Check sheet for the modelled part. Datum: model origin and axes. Units: mm. A direction names the side the tool comes from. Give positions to 0.01 mm unless a question says otherwise; leave off trailing zeros. Loops run counter-clockwise (first coordinate to the right, second up) from the corner with the lowest first, then second, coordinate; pieces in that order, holes last. Notation, with made-up numbers: (22.5, 59.5) -> (78.5, 59.5) arc R32 ccw to (78.5, 91.5) -> close; hole circle Ø5 at (51, -34.75). An arc over 180 degrees is marked (long way). Answer as CSV lines item,"result". Start each with the question number.
(1) Material ranges on line 1 (X direction, y = 14.25, z = 0) (3 decimals); line 2 (Y direction, x = 21.5, z = 2.5); line 3 (Z direction, x = 4, y = 13), recorded low to high. Write a range as from..to.
(2) Section check A-A on z = 0. Enter the section's corners in (x, y) (3 decimals), plus the area to 3 significant figures.
(3) Release check for a two-part mould opening along Z. For faces 6 (the face through (-24, 20, 0)), 7 (the face through (3.3, 0, -3.3)), 8 (the face through (-3.99, 10.5, -2.07)) record: pulls with the +Z half, pulls with the -Z half, needs draft (parallel to the pull), parting line crosses it, or undercut.
(4) Section check D-D on y = 9.75. Enter the section's corners in (x, z) (3 decimals).
(5) Section check C-C on y = 19.5. Enter the section's corners in (x, z) (3 decimals).
(6) Section check B-B on x = 0. Enter the section's corners in (y, z) (3 decimals).
(7) Access from +Z, -Z, +X, -X, +Y, -Y to the whole of each face (thin tool, end or side, straight path). Record for faces 1 (the face through (-0.31, 19.78, -12.17)), 2 (the face through (11.5, 9.15, -2.1)), 3 (the face through (21.25, 19.82, -0.06)), 4 (the face through (0, 5, 36)), 5 (the face through (-2.86, 3.86, 16.3)).
(8) Gauge pin test, flat ends, axial feed: pin 1 Ø4 at (x, y) = (-6.5, 4.5) entering from +Z; pin 2 Ø7.5 at (x, z) = (3, 0) entering from -Y; pin 3 Ø1 at (x, y) = (-9.5, 16.5) entering from -Z; pin 4 Ø3 at (y, z) = (9.5, 12.5) entering from +X. Record the tip position at first contact, or that the pin passes through.
from build123d import *

# Parameters (mm, degrees)
SKETCH1_R           = 14
BOSS_EXTRUDE1_DEPTH = 9.15
SKETCH2_R           = 11.5
BOSS_EXTRUDE2_DEPTH = 9.15
BOSS_EXTRUDE3_DEPTH = 3
CUT_EXTRUDE1_START  = -3.000001
CUT_EXTRUDE1_DEPTH  = 3.000002
CUT_EXTRUDE2_DEPTH  = 36.009855755
SKETCH7_R           = 3
BOSS_EXTRUDE4_DEPTH = 19
SKETCH8_R           = 2.75
BOSS_EXTRUDE5_DEPTH = 17
SKETCH9_R           = 4.495
CUT_EXTRUDE3_DEPTH  = 49.225408241


with BuildPart() as part:
    # Sketch1 → Boss-Extrude1 (new body)
    with BuildSketch(Plane(origin=(0, 0, 0), x_dir=(1, 0, 0), z_dir=(0, 1, 0))):
        with Locations(Location((0, 0, 0), (0, 0, 270))):
            Circle(SKETCH1_R)
    extrude(amount=BOSS_EXTRUDE1_DEPTH)

    # Sketch2 → Boss-Extrude2 (add)
    with BuildSketch(Plane(origin=(0, 9.15, 0), x_dir=(1, 0, 0), z_dir=(0, 1, 0))):
        with Locations(Location((0, 0, 0), (0, 0, 270))):
            Circle(SKETCH2_R)
    extrude(amount=BOSS_EXTRUDE2_DEPTH)

    # Sketch3 → Boss-Extrude3 (add)
    with BuildSketch(Plane(origin=(0, 18.3, 0), x_dir=(1, 0, 0), z_dir=(0, 1, 0))):
        with BuildLine():
            Line((-20.684849103, -12.171155146), (20.684849103, -12.171155146))
            ThreePointArc((20.684849103, -12.171155146), (24, 0), (20.684849103, 12.171155146))
            Line((20.684849103, 12.171155146), (-20.684849103, 12.171155146))
            ThreePointArc((-20.684849103, 12.171155146), (-24, 0), (-20.684849103, -12.171155146))
        make_face()
    extrude(amount=BOSS_EXTRUDE3_DEPTH)

    # Sketch4 → Cut-Extrude1 (cut)
    with BuildSketch(Plane(origin=(0, 21.3, 0), x_dir=(1, 0, 0), z_dir=(0, 1, 0)).offset(CUT_EXTRUDE1_START)):
        with BuildLine():
            Line((-21.82865512, -9.975460673), (-21.82865512, -23.828437081))
            Line((-21.82865512, -23.828437081), (21.82865512, -23.828437081))
            Line((21.82865512, -23.828437081), (21.82865512, -9.975460673))
            ThreePointArc((21.82865512, -9.975460673), (0, -12.171155146), (-21.82865512, -9.975460673))
        make_face()
        with BuildLine():
            Line((21.82865512, 9.975460673), (21.82865512, 24.795204082))
            Line((21.82865512, 24.795204082), (-21.82865512, 24.795204082))
            Line((-21.82865512, 24.795204082), (-21.82865512, 9.975460673))
            ThreePointArc((-21.82865512, 9.975460673), (0, 12.171155146), (21.82865512, 9.975460673))
        make_face()
    extrude(amount=CUT_EXTRUDE1_DEPTH, mode=Mode.SUBTRACT)

    # Sketch6 → Cut-Extrude2 (cut, through all)
    with BuildSketch(Plane(origin=(0, 21.3, 0), x_dir=(1, 0, 0), z_dir=(0, 1, 0))):
        with BuildLine():
            ThreePointArc((-20.773998678, 4.472524896), (-21.25, 0), (-20.773998678, -4.472524896))
            ThreePointArc((-20.773998678, -4.472524896), (-18.100837358, -6.198563297), (-16.374798958, -3.525401977))
            ThreePointArc((-16.374798958, -3.525401977), (-16.75, 0), (-16.374798958, 3.525401977))
            ThreePointArc((-16.374798958, 3.525401977), (-18.100837358, 6.198563297), (-20.773998678, 4.472524896))
        make_face()
    cut_extrude2 = extrude(amount=-CUT_EXTRUDE2_DEPTH, mode=Mode.SUBTRACT)

    # Mirror1: Cut-Extrude2 across plane
    add(cut_extrude2.mirror(Plane(origin=(0, 0, 0), x_dir=(0, 0, 1), z_dir=(1, 0, 0))), mode=Mode.SUBTRACT)

    # Sketch7 → Boss-Extrude4 (add)
    with BuildSketch(Plane.XY):
        with Locations(Location((0, 4.762483919, 0), (0, 0, 180))):
            Circle(SKETCH7_R)
    extrude(amount=BOSS_EXTRUDE4_DEPTH)

    # Sketch8 → Boss-Extrude5 (add)
    with BuildSketch(Plane.XY.offset(19)):
        with Locations((0, 4.762483919)):
            Circle(SKETCH8_R)
    extrude(amount=BOSS_EXTRUDE5_DEPTH)

    # Sketch9 → Cut-Extrude3 (cut, through all)
    with BuildSketch(Plane.XZ):
        with Locations(Location((0, 0, 0), (0, 0, 270))):
            Circle(SKETCH9_R)
    extrude(amount=-CUT_EXTRUDE3_DEPTH, mode=Mode.SUBTRACT)


solid = part.part
Working result:
1,line 1,"x = -11.5..-4.495, 4.495..11.5"
1,line 2,"y = 18.3..21.3"
1,line 3,"z = -10.78..-2.05, 2.05..10.78"
2,outline,"(-24, 18.3) -> (-21.25, 18.3) -> (-21.25, 21.3) -> (-24, 21.3) -> close; (-16.75, 18.3) -> (-11.5, 18.3) -> (-11.5, 9.15) -> (-14, 9.15) -> (-14, 0) -> (-4.495, 0) -> (-4.495, 21.3) -> (-16.75, 21.3) -> close; (4.495, 0) -> (14, 0) -> (14, 9.15) -> (11.5, 9.15) -> (11.5, 18.3) -> (16.75, 18.3) -> (16.75, 21.3) -> (4.495, 21.3) -> close; (21.25, 18.3) -> (24, 18.3) -> (24, 21.3) -> (21.25, 21.3) -> close"
2,area,"392 mm^2"
3,face 6,"parting line crosses it"
3,face 7,"needs draft"
3,face 8,"undercut"
4,outline,"circle Ø23 at (0, 0); hole circle Ø8.99 at (0, 0)"
5,outline,"(-21.829, -9.975) arc R109.603 ccw to (21.829, -9.975) arc R24 ccw to (21.829, 9.975) arc R109.603 ccw to (-21.829, 9.975) arc R24 ccw to start; hole (-20.774, -4.473) arc R2.25 ccw to (-16.375, -3.525) arc R16.75 cw to (-16.375, 3.525) arc R2.25 ccw to (-20.774, 4.473) arc R21.25 ccw to start; hole circle Ø8.99 at (0, 0); hole (16.375, -3.525) arc R2.25 ccw to (20.774, -4.473) arc R21.25 ccw to (20.774, 4.473) arc R2.25 ccw to (16.375, 3.525) arc R16.75 cw to start"
6,outline,"(0, -14) -> (9.15, -14) -> (9.15, -11.5) -> (18.3, -11.5) -> (18.3, -12.171) -> (21.3, -12.171) -> (21.3, -4.495) -> (0, -4.495) -> close; (0, 4.495) -> (21.3, 4.495) -> (21.3, 12.171) -> (18.3, 12.171) -> (18.3, 11.5) -> (9.15, 11.5) -> (9.15, 14) -> (7.762, 14) -> (7.762, 19) -> (7.512, 19) -> (7.512, 36) -> (2.012, 36) -> (2.012, 19) -> (1.762, 19) -> (1.762, 14) -> (0, 14) -> close"
7,face 1,"-Z, +Y"
7,face 2,"none"
7,face 3,"+Y, -Y"
7,face 4,"+Z, +X, -X, +Y, -Y"
7,face 5,"+Z"
8,pin 1,"stops at z = 13.26"
8,pin 2,"stops at y = 0"
8,pin 3,"stops at z = -7.16"
8,pin 4,"stops at x = 8.61"
